The drawing under review shows one solid part. Ordinate dimensions are in mm from its lowest x, y, z. A direction names the side the tool comes from. Coordinates: 2 decimals unless noted, no trailing zeros. Order: outer loops, then holes, each group sorted by start corner. A loop starts at its lowest first (then second) coordinate and runs counter-clockwise, first axis right, second up. Notation, with made-up numbers: M 31,-37.5 L 79,-37.5 A22 cw 79,-6.5 Z; hole C 59,16.5 d2. An arc over 180 degrees is marked long. Answer as a JSON object with one key per item and string values.
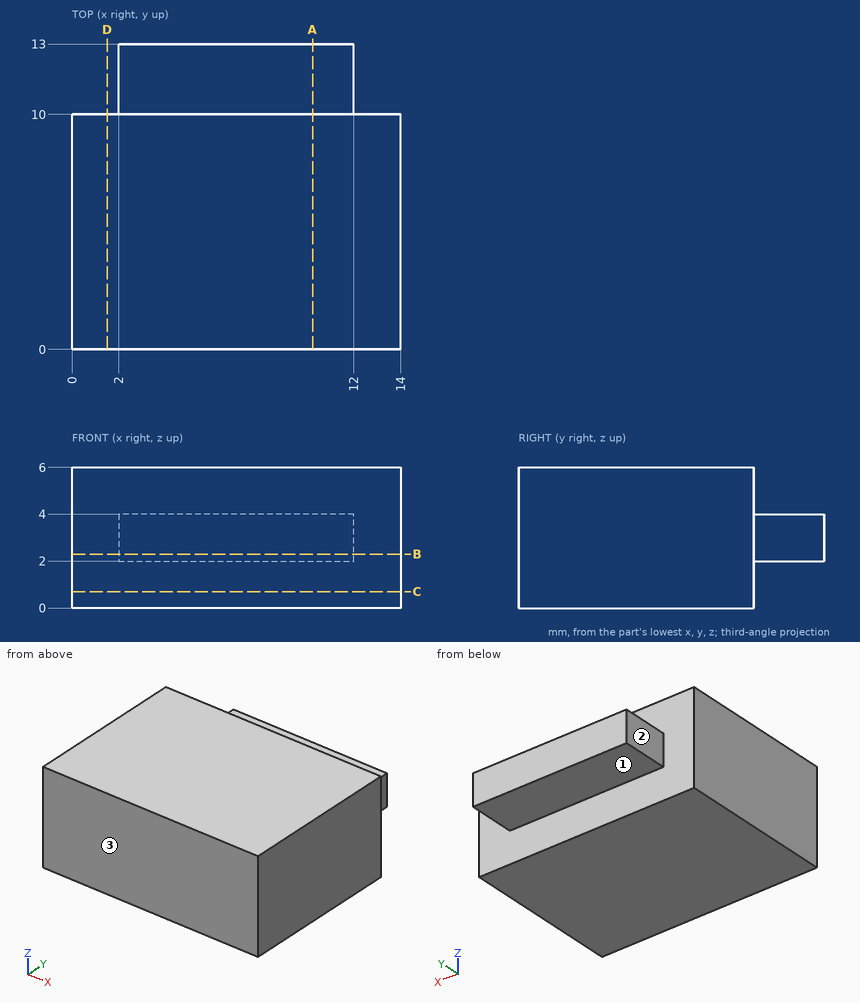
1) Tool access review of the marked faces 1, 2 and 3: name each direction out of +Z, -Z, +X, -X, +Y, -Y from which nothing blocks a thin tool from reaching the whole face with its end or side.
Taken from the geometry:
{"face 1": "-Z, +X, -X, +Y", "face 2": "+Z, -Z, -X, +Y", "face 3": "+Z, -Z, +X, -X, -Y"}
2) Insertion check: pin 1 Ø1.5 at (y, z) = (4.5, 2) entering from -X; pin 2 Ø1 at (y, z) = (11.5, 3) entering from +X; pin 3 Ø1.5 at (x, y) = (6, 11.5) entering from +Z; pin 4 Ø1.6 at (y, z) = (11, 3) entering from -X. Each pin has a flat end and moves straight along its axis. Give the tip position at first contact, or say it passes through.
Taken from the geometry:
{"pin 1": "stops at x = 0", "pin 2": "stops at x = 12", "pin 3": "stops at z = 4", "pin 4": "stops at x = 2"}
3) To check wall thickness, follow L1, parallel to Z at x = 7.25, y = 11.5; L2, parallel to Y at x = 10.25, z = 5.6. State the ranges of each line that lie inside material, in increasing order.
Taken from the geometry:
{"L1": "z = 2 to 4", "L2": "y = 0 to 10"}
4) Add section C-C (z = 0.7). State the section outline as (x, y) points, and give its area (3 significant figures).
Taken from the geometry:
{"outline": "M 0,0 L 14,0 L 14,10 L 0,10 Z", "area": "140 mm2"}
5) Add section B-B (z = 2.3). State the section outline as (x, y) points, and give its area (3 significant figures).
Taken from the geometry:
{"outline": "M 0,0 L 14,0 L 14,10 L 12,10 L 12,13 L 2,13 L 2,10 L 0,10 Z", "area": "170 mm2"}
6) Add section D-D (x = 1.5). State the section outline as (y, z) points, and give its area (3 significant figures).
Taken from the geometry:
{"outline": "M 0,0 L 10,0 L 10,6 L 0,6 Z", "area": "60.0 mm2"}
7) Add section A-A (x = 10.25). State the section outline as (y, z) points.
Taken from the geometry:
{"outline": "M 0,0 L 10,0 L 10,2 L 13,2 L 13,4 L 10,4 L 10,6 L 0,6 Z"}
